```python
from build123d import *

# Parameters (mm, degrees)
SKETCH1_W           = 11.695168442
SKETCH1_H           = 12.807944464
BOSS_EXTRUDE1_DEPTH = 2


with BuildPart() as part:
    # Sketch1 → Boss-Extrude1 (new body)
    with BuildSketch(Plane.XY):
        Polygon((0, 0), (35, 0), (35, -2.000471596), (80.41, -2.000471596), (80.41, 0), (115.41, 0), (115.41, 5), (117.41, 5), (117.41, 15), (115.409999943, 15), (115.409999943, 20.003619975), (81.929720774, 20.003619975), (81.929720774, 4.189216968), (68.473093168, 4.189216968), (68.473093168, 15.598586388), (68.473093168, 19.951067772), (68.473093168, 22), (35, 22), (35, 20), (0, 20), (0, 15), (-2, 15), (-2, 5), (0, 5), align=None)
        with Locations((15.847584221, 11.403972232)):
            Rectangle(SKETCH1_W, SKETCH1_H, mode=Mode.SUBTRACT)
    extrude(amount=BOSS_EXTRUDE1_DEPTH)


solid = part.part
```
Verification items for the finished model (mm, model axes). A direction names the side the tool comes from. Coordinates: 2 decimals unless noted, no trailing zeros. Loops run counter-clockwise (first coordinate to the right, second up) from the corner with the lowest first, then second, coordinate; pieces in that order, holes last. Notation, with made-up numbers: (70.5, 65) -> (128.5, 65) arc R31 cw to (128.5, 97) -> close; hole circle Ø7 at (18.25, 8). An arc over 180 degrees is marked (long way). Answer in a Markdown table with one row per item.
1) Draft check along Y on faces 1 (the face through (-1, 5, 1)), 2 (the face through (16, 5, 1)), 3 (the face through (57, 10, 2)). Enter one of: released by +Y, released by -Y, zero draft, split by the parting line, or undercut.
The answers:
| item | result |
|---|---|
| face 1 | released by -Y |
| face 2 | undercut |
| face 3 | zero draft |
2) Section check C-C (x = 30). Record the cut outline in (y, z).
The answers:
| item | result |
|---|---|
| outline | (0, 0) -> (20, 0) -> (20, 2) -> (0, 2) -> close |
3) Section check B-B (z = 1.1). Record the cut outline in (x, y).
The answers:
| item | result |
|---|---|
| outline | (-2, 5) -> (0, 5) -> (0, 0) -> (35, 0) -> (35, -2) -> (80.41, -2) -> (80.41, 0) -> (115.41, 0) -> (115.41, 5) -> (117.41, 5) -> (117.41, 15) -> (115.41, 15) -> (115.41, 20) -> (81.93, 20) -> (81.93, 4.19) -> (68.47, 4.19) -> (68.47, 22) -> (35, 22) -> (35, 20) -> (0, 20) -> (0, 15) -> (-2, 15) -> close; hole (10, 5) -> (21.7, 5) -> (21.7, 17.81) -> (10, 17.81) -> close |
4) Section check A-A (y = 13.5). Record the cut outline in (x, z).
The answers:
| item | result |
|---|---|
| outline | (-2, 0) -> (10, 0) -> (10, 2) -> (-2, 2) -> close; (21.7, 0) -> (68.47, 0) -> (68.47, 2) -> (21.7, 2) -> close; (81.93, 0) -> (117.41, 0) -> (117.41, 2) -> (81.93, 2) -> close |
5) Scan lines: line 1 along X through (y, z) = (7, 1.3); line 2 along X through (y, z) = (15.75, 1); line 3 along X through (y, z) = (18, 1.85). Record each from-to range of solid material in increasing order. Write a range as from..to.
The answers:
| item | result |
|---|---|
| line 1 | x = -2..10, 21.7..68.47, 81.93..117.41 |
| line 2 | x = 0..10, 21.7..68.47, 81.93..115.41 |
| line 3 | x = 0..68.47, 81.93..115.41 |
6) Access from +Z, -Z, +X, -X, +Y, -Y to the whole of each face (thin tool, end or side, straight path). Record for faces 4 (the face through (35, -1, 1)), 5 (the face through (99, 20.004, 1)), 6 (the face through (10, 11, 1)).
The answers:
| item | result |
|---|---|
| face 4 | +Z, -Z, -X, -Y |
| face 5 | +Z, -Z, +X, +Y |
| face 6 | +Z, -Z |
7) Depth check by flat-ended pin: P1, Ø0.6, axis at y = 1.5, z = 1, coming from the +X side; P2, Ø0.6, axis at x = -1, z = 0.5, coming from the -Y side; P3, Ø1, axis at y = 17, z = 1, coming from the -X side. Enter the tip coordinate at first touch or a pass-through.
The answers:
| item | result |
|---|---|
| P1 | stops at x = 115.41 |
| P2 | stops at y = 5 |
| P3 | stops at x = 0 |
